Read the model definition and answer for the solid it produces. Units are mm, in the model's axes. A direction names the side the tool comes from. Round coordinates to 2 decimals unless told otherwise and drop trailing zeros. Order: outer loops, then holes, each group sorted by start corner. A loop starts at its lowest first (then second) coordinate and runs counter-clockwise, first axis right, second up. Notation, with made-up numbers: (-5.75, 62.5) -> (43.25, 62.5) arc R29 cw to (43.25, 93.5) -> close; hole circle Ø10 at (80.5, -34). An arc over 180 degrees is marked (long way). Answer as a JSON object with one key per item and string values. Group by question number.
Item 1: For faces 4 (the cylindrical face through (-5.35, 2.95, -3.09)), 5 (the flat face through (-1, 7.956, 0)), determine the directions among +Z, -Z, +X, -X, +Y, -Y from which every point of the face is accessible in a straight line to the end or side of a thin tool.
Item 2: Consider probe 1 along X at (y, z) = (4.75, 0); probe 2 along X at (y, z) = (7.75, 0); probe 3 along Y at (x, z) = (-1.5, 2). Determine where each line is inside the solid, lowest interval first. Write a range as from..to.
Item 3: Given P1, Ø1, axis at x = 2, y = 4, coming from the +Z side; P2, Ø1, axis at y = 5.5, z = 2.5, coming from the +X side; P3, Ø5, axis at x = 0, z = 0.5, coming from the -Y side, each flat-ended and moving along its own axis, determine where each tip first touches the part or whether it passes through.
Item 4: Section A-A, the plane y = 6.75 is taken. Write down the section's boundary in (x, z), plus the area to 3 significant figures.
Item 5: The mould has two halves that part along X. Classify faces 1 (the flat face through (-5, 3.978, -2)), 2 (the cylindrical face through (4.137, 7.227, 1.03)), 3 (the cylindrical face through (4.137, 4.717, 1.03)): pulls with the +X half, pulls with the -X half, needs draft (parallel to the pull), parting line crosses it, or undercut.
from build123d import *

# Parameters (mm, degrees)
FILLET1_R = 2
FILLET2_R = 2
FILLET3_R = 2
FILLET4_R = 1


with BuildPart() as part:
    # Sketch1 → Revolve1 (revolve)
    with BuildSketch(Plane.XY, mode=Mode.PRIVATE) as revolve1_sk:
        Polygon((-0.5, 8.956259778), (-6.25, 8.956259778), (-6.25, 5.477980263), (-5.25, 5.477980263), (-5.25, 3.977980263), (-6.25, 3.977980263), (-6.25, 1.956259778), (-5.25, 1.956259778), (-5.25, 2.977980263), (-4.25, 2.977980263), (-4.25, 6.477980263), (-5.25, 6.477980263), (-5.25, 7.956259778), (-0.5, 7.956259778), align=None)
    revolve(revolve1_sk.sketch.rotate(Axis((-0.5, 1.956259778, 0), (0, 1, 0)), 270), axis=Axis((-0.5, 1.956259778, 0), (0, 1, 0)))

    # Fillet1
    # the kernel refuses this fillet: 2 mm, written as the material it takes off along each edge
    with BuildSketch(Plane(origin=(-0.5, 2.977980263, 0), x_dir=(0, 0, -1), z_dir=(1, 0, 0))) as fillet1_piece_1:
        with BuildLine():
            CenterArc((5.75, 1.732050808), FILLET1_R, 180, 60)
            Line((3.75, 1.732050808), (3.71, 1.732050808))
            Line((3.71, 1.732050808), (3.71, 0))
            Line((3.71, 0), (3.75, -0.04))
            ThreePointArc((3.75, -0.04), (4.25, -0.04), (4.73, -0.034641016))
            Line((4.73, -0.034641016), (4.75, 0))
        make_face()
    revolve(axis=Axis((-0.5, 2.977980263, 0), (0, 1, 0)), mode=Mode.SUBTRACT)

    # Fillet2
    fillet2_edges = [part.edges().sort_by_distance(p)[0] for p in [
        (-0.5, 2.977980263, 4.75),
    ]]
    fillet(fillet2_edges, radius=FILLET2_R)

    # Fillet3
    # the kernel refuses this fillet: 2 mm, written as the material it takes off along each edge
    with BuildSketch(Plane(origin=(-0.5, 6.477980263, 0), x_dir=(0, 0, -1), z_dir=(1, 0, 0))) as fillet3_piece_1:
        with BuildLine():
            CenterArc((5.75, -1.732050808), FILLET3_R, 120, 60)
            Line((4.75, 0), (4.73, 0.034641016))
            ThreePointArc((4.73, 0.034641016), (4.25, 0.04), (3.75, 0.04))
            Line((3.75, 0.04), (3.71, 0))
            Line((3.71, 0), (3.71, -1.732050808))
            Line((3.71, -1.732050808), (3.75, -1.732050808))
        make_face()
    revolve(axis=Axis((-0.5, 6.477980263, 0), (0, 1, 0)), mode=Mode.SUBTRACT)

    # Fillet4
    fillet4_edges = [part.edges().sort_by_distance(p)[0] for p in [
        (-0.5, 8.956259778, 5.75),
    ]]
    fillet(fillet4_edges, radius=FILLET4_R)


solid = part.part
Values found:
{
 "1": {"face 4": "+Y, -Y", "face 5": "none"},
 "2": {"probe 1": "-5.25..-4.25, 3.25..4.25", "probe 2": "-6.25..-5.25, 4.25..5.25", "probe 3": "7.96..8.96"},
 "3": {"P1": "z = 5.39", "P2": "x = 4.89", "P3": "y = 7.96"},
 "4": {"outline": "circle Ø11.5 at (-0.5, 0); hole circle Ø9.5 at (-0.5, 0)", "area": "33.0 mm2"},
 "5": {"face 1": "needs draft", "face 2": "undercut", "face 3": "parting line crosses it"}
}
